from build123d import *

# Parameters (mm, degrees)
SKETCH_1_W             = 40
SKETCH_1_H             = 40
EXTRUDE_1_DEPTH        = 500
EXTRUDE_1_2_DEPTH      = 500
EXTRUDE_1_3_DEPTH      = 500
EXTRUDE_1_4_DEPTH      = 500
SKETCH_3_W             = 40
SKETCH_3_H             = 440
EXTRUDE_2_DEPTH        = 40
SKETCH_4_W             = 40
SKETCH_4_H             = 440
EXTRUDE_3_DEPTH        = 40
SKETCH_5_W             = 40
SKETCH_5_H             = 40
EXTRUDE_4_DEPTH        = 100
EXTRUDE_5_DEPTH        = 40
EXTRUDE_6_DEPTH        = 40
EXTRUDE_7_DEPTH        = 40
PATTERN_LINEAR_1_COUNT = 2
PATTERN_LINEAR_1_PITCH = 100
EXTRUDE_8_DEPTH        = 40
EXTRUDE_9_DEPTH        = 40


with BuildPart() as part:
    # Sketch 1 → Extrude 1 (new body)
    with BuildSketch(Plane(origin=(0, 0, 0), x_dir=(1, 0, 0), z_dir=(0, 1, 0))):
        with Locations((20, -20)):
            Rectangle(SKETCH_1_W, SKETCH_1_H)
    extrude(amount=EXTRUDE_1_DEPTH)



with BuildPart() as body_2:
    # Sketch 1 → Extrude 1 2 (new body)
    with BuildSketch(Plane(origin=(0, 0, 0), x_dir=(1, 0, 0), z_dir=(0, 1, 0))):
        with Locations((120, -20)):
            Rectangle(SKETCH_1_W, SKETCH_1_H)
    extrude(amount=EXTRUDE_1_2_DEPTH)



with BuildPart() as body_3:
    # Sketch 1 → Extrude 1 3 (new body)
    with BuildSketch(Plane(origin=(0, 0, 0), x_dir=(1, 0, 0), z_dir=(0, 1, 0))):
        with Locations((20, -120)):
            Rectangle(SKETCH_1_W, SKETCH_1_H)
    extrude(amount=EXTRUDE_1_3_DEPTH)


with BuildPart() as body_4:
    # Sketch 1 → Extrude 1 4 (new body)
    with BuildSketch(Plane(origin=(0, 0, 0), x_dir=(1, 0, 0), z_dir=(0, 1, 0))):
        with Locations((120, -120)):
            Rectangle(SKETCH_1_W, SKETCH_1_H)
    extrude(amount=EXTRUDE_1_4_DEPTH)


with BuildPart() as part_1:
    add(part.part)

    add(body_3.part)  # Extrude 2 merges body 3
    # Sketch 3 → Extrude 2 (add)
    with BuildSketch(Plane(origin=(0, 500, 0), x_dir=(1, 0, 0), z_dir=(0, 1, 0))):
        with Locations((20, -70)):
            Rectangle(SKETCH_3_W, SKETCH_3_H)
    extrude(amount=EXTRUDE_2_DEPTH)



with BuildPart() as body_2_1:
    add(body_2.part)

    add(body_4.part)  # Extrude 3 merges body 4
    # Sketch 4 → Extrude 3 (add)
    with BuildSketch(Plane(origin=(0, 500, 0), x_dir=(1, 0, 0), z_dir=(0, 1, 0))):
        with Locations((120, -70)):
            Rectangle(SKETCH_4_W, SKETCH_4_H)
    extrude(amount=EXTRUDE_3_DEPTH)


with BuildPart() as part_2:
    add(part_1.part)

    add(body_2_1.part)  # Extrude 4 merges body 2
    # Sketch 5 → Extrude 4 (add)
    with BuildSketch(Plane(origin=(40, 0, 0), x_dir=(0, 0, -1), z_dir=(1, 0, 0))):
        with Locations((-120, 520)):
            Rectangle(SKETCH_5_W, SKETCH_5_H)
        with Locations((-20, 520)):
            Rectangle(SKETCH_5_W, SKETCH_5_H)
    extrude(amount=EXTRUDE_4_DEPTH)

    # Sketch 6 → Extrude 5 (add)
    with BuildSketch(Plane(origin=(140, 0, 0), x_dir=(0, 0, -1), z_dir=(1, 0, 0))):
        Polygon((-290, 500), (-140, 350), (-140, 406.568542495), (-233.431457505, 500), align=None)
        Polygon((150, 500), (0, 350), (0, 406.568542495), (93.431457505, 500), align=None)
    extrude(amount=-EXTRUDE_5_DEPTH)

    # Sketch 7 → Extrude 6 (add)
    with BuildSketch(Plane.ZY):
        Polygon((-150, 500), (0, 350), (0, 406.568542495), (-93.431457505, 500), align=None)
        Polygon((290, 500), (140, 350), (140, 413.639610307), (226.360389693, 500), align=None)
    extrude(amount=-EXTRUDE_6_DEPTH)

    # Sketch 8 → Extrude 7 (add)
    with BuildSketch(Plane.ZY):
        Polygon((0, 143.431457505), (0, 200), (-200, 0), (-143.431457505, 0), align=None)
        Polygon((140, 143.431457505), (283.431457505, 0), (340, 0), (140, 200), align=None)
    extrude_7 = extrude(amount=-EXTRUDE_7_DEPTH)

    # Pattern Linear 1: Extrude 7 ×2
    with Locations(*[(i * PATTERN_LINEAR_1_PITCH, 0, 0) for i in range(1, PATTERN_LINEAR_1_COUNT)]):
        add(extrude_7)

    # Sketch 9 → Extrude 8 (add)
    with BuildSketch(Plane(origin=(0, 0, 0), x_dir=(-1, 0, 0), z_dir=(0, 0, -1))):
        Polygon((-340, 0), (-283.431457505, 0), (-140, 143.431457505), (-140, 200), align=None)
        Polygon((200, 0), (0, 200), (0, 143.431457505), (143.431457505, 0), align=None)
    extrude(amount=-EXTRUDE_8_DEPTH)

    # Sketch 10 → Extrude 9 (add)
    with BuildSketch(Plane.XY.offset(140)):
        Polygon((0, 143.431457505), (0, 200), (-200, 0), (-143.431457505, 0), align=None)
        Polygon((140, 143.431457505), (283.431457505, 0), (340, 0), (140, 200), align=None)
    extrude(amount=-EXTRUDE_9_DEPTH)


solid = part_2.part
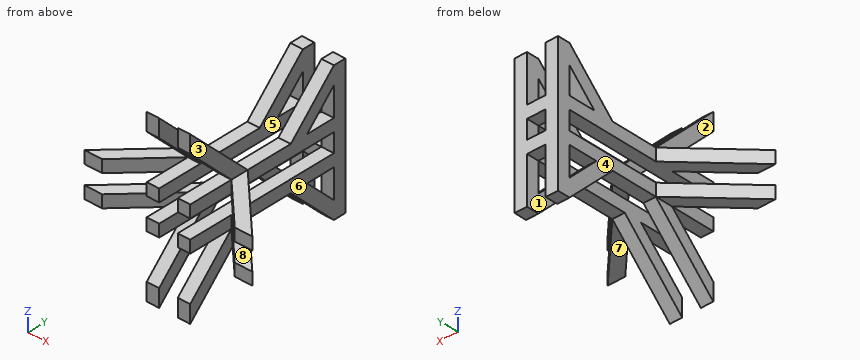
Input: part model. Units: mm. Frame: model coordinates. Face numbers are marked on the shaded views. A direction names the side the tool comes from. Give positions to 0.01 mm unless a question says otherwise; leave off trailing zeros. Write each loop counter-clockwise with the first axis right and the second up, starting at its lowest first coordinate (ties: lowest second). Pieces come first, ordered by that corner, then holes.
Q1. Set-up query: the marked faces 1, 2, 3, 4 and 5. Return all of +Z, -Z, +X, -X, +Y, -Y with unobstructed straight access to the full face (end or side cutting, diameter ignored); none if empty.
Q2. Section C-C, the plane x = 68. Output: boundary loops of the cut face in (y, z).
Q3. Material intervals for probe 1 along X at (y, z) = (104, 38); probe 2 along X at (y, z) = (128, -68.5), sorted ascending.
Q4. Section A-A, the plane z = 77. Output: boundary loops of the cut face in (x, y), plus the area to 3 significant figures.
Q5. Section B-B, the plane y = 361.5. Output: boundary loops of the cut face in (x, z).
Q6. Pull-direction query (Z, two-part tool) for the marked faces 6, 7 and 8; classes: pulls with the +Z half, pulls with the -Z half, needs draft (parallel to the pull), parting line crosses it, or undercut.
Q7. Section D-D, the plane z = -54.5. Output: boundary loops of the cut face in (x, y).
Q8. First-contact query: P1, Ø1.5, axis at x = 12, z = 97.5, coming from the -Y side; P2, Ø20, axis at x = 121.5, z = -67, coming from the -Y side; P3, Ø20, axis at x = 59.5, y = 524.5, coming from the -Z side. Flat tips, straight axial feed; report the tip coordinate or a pass-through.
Filled in:
1. face 1: -Z, -Y
1. face 2: +Z, -X, +Y, -Y
1. face 3: +Z, +X, +Y, -Y
1. face 4: +Z, -Z, -X, +Y
1. face 5: +Z, -Y
2. outline: (500, 0) - (540, 0) - (540, 40) - (500, 40) - close; (500, 100) - (540, 100) - (540, 140) - (500, 140) - close
3. probe 1: x = -96 to -39.43, 0 to 40, 100 to 140, 179.43 to 236
3. probe 2: x = 0 to 40, 100 to 140
4. outline: (0, 500) - (40, 500) - (40, 540) - (0, 540) - close; (100, 500) - (140, 500) - (140, 540) - (100, 540) - close
4. area: 3,200 mm2
5. outline: (0, -11.5) - (40, -11.5) - (40, 40) - (0, 40) - close; (0, 100) - (40, 100) - (40, 151.5) - (0, 151.5) - close; (100, -11.5) - (140, -11.5) - (140, 40) - (100, 40) - close; (100, 100) - (140, 100) - (140, 151.5) - (100, 151.5) - close
6. face 6: needs draft
6. face 7: pulls with the -Z half
6. face 8: undercut
7. outline: (0, 88.93) - (40, 88.93) - (40, 145.5) - (0, 145.5) - close; (0, 404.5) - (40, 404.5) - (40, 461.07) - (0, 461.07) - close; (0, 500) - (40, 500) - (40, 540) - (0, 540) - close; (100, 88.93) - (140, 88.93) - (140, 145.5) - (100, 145.5) - close; (100, 404.5) - (140, 404.5) - (140, 461.07) - (100, 461.07) - close; (100, 500) - (140, 500) - (140, 540) - (100, 540) - close
8. P1: stops at y = 500
8. P2: stops at y = 66.43
8. P3: stops at z = 0
